```python
from build123d import *

# Parameters (mm, degrees)
F0_W   = 1.5875
F0_H   = 15.875
F0_W_2 = 11.1125
F0_H_2 = 69.85


# Not quite as in the source:
# - a fillet or chamfer that OpenCascade refuses, or shapes differently, is made with other operations: its cross-section is extruded or revolved along the edge and cut away or added


with BuildPart() as f1:
    # F0 (on Front) → F1 (revolve)
    with BuildSketch(Plane.XZ):
        with Locations((-11.90625, 217.4875)):
            Rectangle(F0_W, F0_H)
        with Locations((-5.55625, 217.4875)):
            Rectangle(F0_W_2, F0_H)
        with Locations((-5.55625, 174.625)):
            Rectangle(F0_W_2, F0_H_2)
        with BuildLine():
            Line((-38.1, 101.6), (0, 101.6))
            Line((0, 101.6), (0, 139.7))
            Line((0, 139.7), (-11.1125, 139.7))
            ThreePointArc((-11.1125, 139.7), (-14.586457312, 129.203622534), (-23.4018713236, 122.5304827094))
            ThreePointArc((-23.4018713236, 122.5304827094), (-34.0584362623, 114.387885801), (-38.1, 101.6))
        make_face()
        with BuildLine():
            Line((0, -85.043540958), (0, 101.6))
            Line((0, 101.6), (-38.1, 101.6))
            Line((-38.1, 101.6), (-38.1, -101.6))
            Line((-38.1, -101.6), (-24.4468970238, -101.6))
            ThreePointArc((-24.4468970238, -101.6), (-18.8855290947, -99.8940128678), (-15.2374166451, -95.3629554974))
            ThreePointArc((-15.2374166451, -95.3629554974), (-9.2014833377, -87.8661580499), (0, -85.043540958))
        make_face()
    revolve(axis=Axis((0, 0, 70.190729521), (0, 0, 1)))

    # F2: fillet of radius 3.175 on 3 edges, made by hand

    # F2_s1 → F2_t2 (revolve, cut)
    with BuildSketch(Plane.XZ):
        with BuildLine():
            ThreePointArc((-38.1, -98.425), (-37.1700640303, -100.6700640303), (-34.925, -101.6))
            Line((-34.925, -101.6), (-34.925, -101.6635))
            Line((-34.925, -101.6635), (-38.1635, -101.6635))
            Line((-38.1635, -101.6635), (-38.1635, -98.425))
            Line((-38.1635, -98.425), (-38.1, -98.425))
        make_face()
    revolve(axis=Axis((0, 0, -101.6), (0, 0, 1)), mode=Mode.SUBTRACT)

    # F2_s3 → F2_t4 (revolve, cut)
    with BuildSketch(Plane.XZ):
        with BuildLine():
            ThreePointArc((-9.525, 225.425), (-11.7700640303, 224.4950640303), (-12.7, 222.25))
            Line((-12.7, 222.25), (-12.7635, 222.25))
            Line((-12.7635, 222.25), (-12.7635, 225.4885))
            Line((-12.7635, 225.4885), (-9.525, 225.4885))
            Line((-9.525, 225.4885), (-9.525, 225.425))
        make_face()
    revolve(axis=Axis((0, 0, 225.425), (0, 0, 1)), mode=Mode.SUBTRACT)

    # F2_s5 → F2_t6 (revolve, cut)
    with BuildSketch(Plane.XZ):
        with BuildLine():
            ThreePointArc((-11.1125, 209.55), (-12.274630657, 210.712130657), (-12.7, 212.299630657))
            Line((-12.7, 212.299630657), (-12.7635, 212.299630657))
            Line((-12.7635, 212.299630657), (-12.7635, 209.55))
            Line((-12.7635, 209.55), (-12.7, 209.4865))
            ThreePointArc((-12.7, 209.4865), (-11.90625, 209.4865), (-11.14425, 209.4950073869))
            Line((-11.14425, 209.4950073869), (-11.1125, 209.55))
        make_face()
    revolve(axis=Axis((0, 0, 209.55), (0, 0, 1)), mode=Mode.SUBTRACT)


solid = f1.part
```
Check sheet for the modelled part. Datum: model origin and axes. Units: mm. Give positions to 0.01 mm unless a question says otherwise; leave off trailing zeros. Order: outer loops, then holes, each group sorted by start corner. A loop starts at its lowest first (then second) coordinate and runs counter-clockwise, first axis right, second up. Notation, with made-up numbers: M 8.25,46.5 L 63.25,46.5 A21 cw 63.25,68.5 Z; hole C -20,63 d8. An arc over 180 degrees is marked long. Answer in a Markdown table with one row per item. Add a question column.
Q1. Gauge pin test, flat ends, axial feed: pin 1 Ø10 at (x, y) = (12, -20.5) entering from +Z; pin 2 Ø5 at (x, y) = (26, 12) entering from +Z; pin 3 Ø1 at (x, z) = (-12.5, 15) entering from -Y. Record the tip position at first contact, or that the pin passes through.
Q2. Thickness scan on L1, parallel to Y at x = 2, z = -64; L2, parallel to Z at x = -23, y = -14.5; L3, parallel to Z at x = -18.5, y = -7. Record the ranges inside material, lowest first.
Q3. Release check for a two-part mould opening along Z. For faces 1 (the cylindrical face through (2.75, 12.4, 217.34)), 2 (the flat face through (-7, -24, -101.6)), 3 (the cylindrical face through (-10.6, -3.34, 175.11)) record: released by +Z, released by -Z, zero draft, split by the parting line, or undercut.
Q4. Sectioned sample at A-A, the plane z = -72.5. Record the boundary of the cut face in (x, y).
Q5. Sectioned sample at B-B, the plane z = 155.5. Record the boundary of the cut face in (x, y) (1 decimal).
Verdict:
| question | item | result |
|---|---|---|
| 1 | pin 1 | z = 125 |
| 1 | pin 2 | z = 121.33 |
| 1 | pin 3 | y = -36.16 |
| 2 | L1 | -38.05 to 38.05 |
| 2 | L2 | -101.6 to 120.74 |
| 2 | L3 | -100.43 to 124.3 |
| 3 | face 1 | zero draft |
| 3 | face 2 | released by -Z |
| 3 | face 3 | undercut |
| 4 | outline | C 0,0 d76.2 |
| 5 | outline | C 0,0 d22.2 |
